from build123d import *

# Parameters (mm, degrees)
SKETCH_1_W         = 130
SKETCH_1_H         = 250
SKETCH_1_R         = 40
EXTRUDE_1_DEPTH    = 2
HOLE_WIZARD_M4_1_D = 4.5
MIRROR_2_COPY_1_D  = 4.5


with BuildPart() as part:
    # 草图1 → 凸台-拉伸1 (new body)
    with BuildSketch(Plane(origin=(0, 0, 0), x_dir=(1, 0, 0), z_dir=(0, 1, 0))):
        Rectangle(SKETCH_1_W, SKETCH_1_H)
        with Locations(Location((0, 40, 0), (0, 0, 270))):
            Circle(SKETCH_1_R, mode=Mode.SUBTRACT)
    extrude(amount=EXTRUDE_1_DEPTH)

    # M4 间隙孔1 (through all)
    with Locations(Plane(origin=(0, 2, 0), x_dir=(1, 0, 0), z_dir=(0, 1, 0))):
        with Locations((-55, -110), (-55, -33.5)):
            hole_wizard_m4_1 = Hole(HOLE_WIZARD_M4_1_D / 2)

    # 镜向1: M4 间隙孔1 across plane
    add(hole_wizard_m4_1.mirror(Plane.XY), mode=Mode.SUBTRACT)

    # 镜向2: M4 间隙孔1 across plane
    add(hole_wizard_m4_1.mirror(Plane.ZY), mode=Mode.SUBTRACT)

    # 镜向2 copy 1 (through all)
    with Locations(Plane(origin=(0, 2, 0), x_dir=(-1, 0, 0), z_dir=(0, 1, 0))):
        with Locations((-55, -110), (-55, -33.5)):
            Hole(MIRROR_2_COPY_1_D / 2)


solid = part.part
Design review of the part built by this model. Coordinates are the model's own, in mm. Round coordinates to 2 decimals unless told otherwise and drop trailing zeros. Order: outer loops, then holes, each group sorted by start corner. A loop starts at its lowest first (then second) coordinate and runs counter-clockwise, first axis right, second up.
1) Consider section A-A (x = -11). State the section outline as (y, z) points.
The answers:
outline: (0, -125) - (2, -125) - (2, -78.46) - (0, -78.46) - close; (0, -1.54) - (2, -1.54) - (2, 125) - (0, 125) - close
2) Draft analysis for pull direction X (two halves, no side actions). For faces 1 (the flat face through (-15, 0, -2)), 2 (the cylindrical face through (-52.752, 0.986, 33.401)), 3 (the cylindrical face through (54.512, 0.986, 112.196)), state which applies: released by +X, released by -X, zero draft, split by the parting line, or undercut.
The answers:
face 1: zero draft
face 2: undercut
face 3: undercut
3) For L1, parallel to Z at x = 55, y = 1.15; L2, parallel to Z at x = -0.5, y = 0.5; L3, parallel to X at y = 1.4, z = -22, list the stretches that pass through material, from the lowest coordinate up.
The answers:
L1: z = -125 to -112.25, -107.75 to -35.75, -31.25 to 31.25, 35.75 to 107.75, 112.25 to 125
L2: z = -125 to -80, 0 to 125
L3: x = -65 to -35.72, 35.72 to 65
4) Consider section B-B (z = -24.5). State the section outline as (x, y) points.
The answers:
outline: (-65, 0) - (-36.87, 0) - (-36.87, 2) - (-65, 2) - close; (36.87, 0) - (65, 0) - (65, 2) - (36.87, 2) - close
5) Clearance check with a flat-ended pin moving along its axis: pin 1 Ø12 at (x, z) = (-16.5, -68.5) entering from +Y. State where the tip first meets the part, or that it passes through.
The answers:
pin 1: passes through
